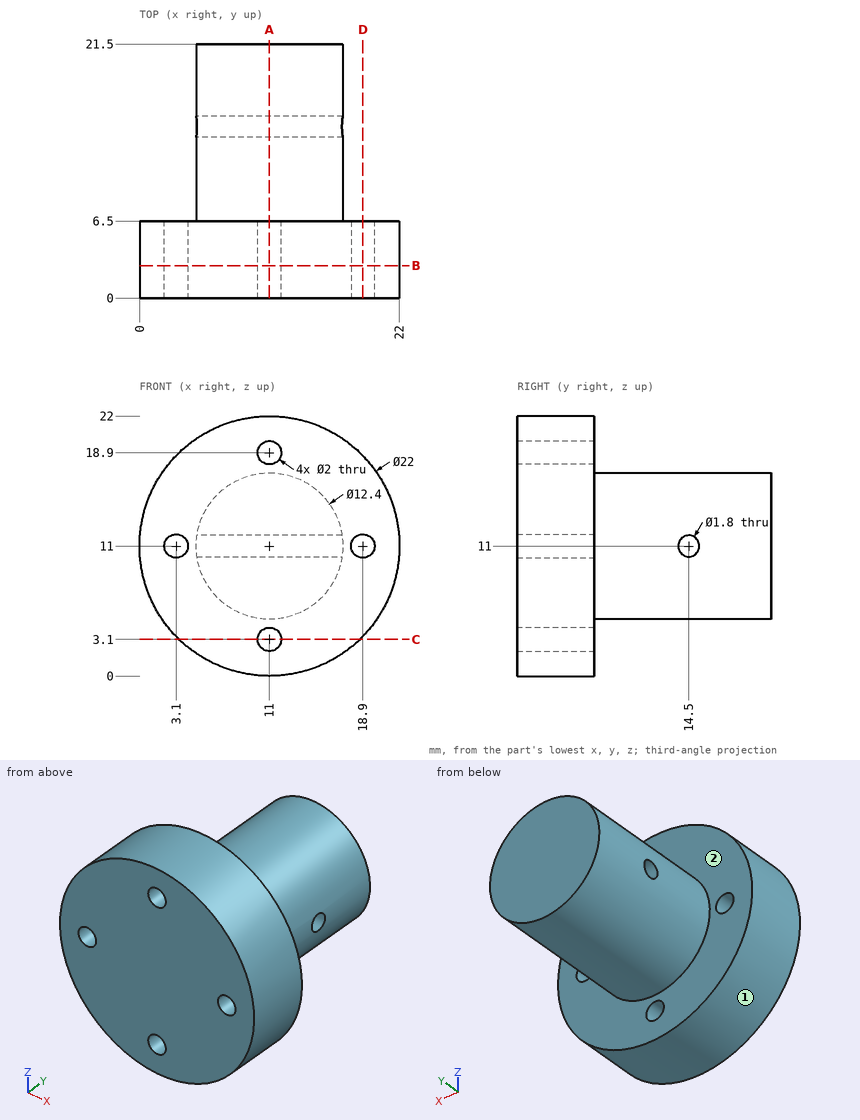
Design review of the part shown in the three views and the two pictorial views. Dimensions are in mm from the part's minimum x, y and z. A direction names the side the tool comes from. Round coordinates to 2 decimals unless told otherwise and drop trailing zeros. Order: outer loops, then holes, each group sorted by start corner. A loop starts at its lowest first (then second) coordinate and runs counter-clockwise, first axis right, second up.
Q1. We need section B-B, the plane y = 2.75. Give the boundary of the cut face in (x, z).
Findings below:
outline: circle Ø22 at (11, 11); hole circle Ø2 at (3.1, 11); hole circle Ø2 at (11, 3.1); hole circle Ø2 at (11, 18.9); hole circle Ø2 at (18.9, 11)
Q2. We need section A-A, the plane x = 11. Give the boundary of the cut face in (y, z), plus the area to 3 significant figures.
Findings below:
outline: (0, 0) - (6.5, 0) - (6.5, 2.1) - (0, 2.1) - close; (0, 4.1) - (6.5, 4.1) - (6.5, 4.8) - (21.5, 4.8) - (21.5, 17.2) - (6.5, 17.2) - (6.5, 17.9) - (0, 17.9) - close; (0, 19.9) - (6.5, 19.9) - (6.5, 22) - (0, 22) - close; hole circle Ø1.8 at (14.5, 11)
area: 300 mm2
Q3. Wall thickness on line 1 (Z direction, x = 10.75, y = 14.5); line 2 (Y direction, x = 6.25, z = 11); line 3 (Y direction, x = 13.75, z = 17.5): over which ranges is each line inside the solid? List them lowest first.
Findings below:
line 1: z = 4.81 to 10.1, 11.9 to 17.19
line 2: y = 0 to 13.6, 15.4 to 21.5
line 3: y = 0 to 6.5
Q4. Insertion check: P1, Ø10, axis at x = 5.5, y = 6, coming from the -Z side; P2, Ø1, axis at x = 10.5, y = 5, coming from the +Z side; P3, Ø4, axis at x = 17.5, y = 17, coming from the +Z side (3 decimals); P4, Ø1.6, axis at y = 14.5, z = 11, coming from the +X side. Each pin has a flat end and moves straight along its axis. Give the tip position at first contact, or say it passes through.
Findings below:
P1: stops at z = 0.01
P2: stops at z = 22
P3: stops at z = 15.265
P4: passes through
Q5. Machinability: for the marked faces 1 and 2, which of the approach directions +Z, -Z, +X, -X, +Y, -Y give a long, thin tool a straight path to every point of the face, cutting with its end or side? Answer none if there is none.
Findings below:
face 1: +Y, -Y
face 2: +Y
Q6. We need section C-C, the plane z = 3.1. Give the boundary of the cut face in (x, y), plus the area to 3 significant figures.
Findings below:
outline: (3.35, 0) - (10, 0) - (10, 6.5) - (3.35, 6.5) - close; (12, 0) - (18.65, 0) - (18.65, 6.5) - (12, 6.5) - close
area: 86.5 mm2
Q7. We need section D-D, the plane x = 18.9. Give the boundary of the cut face in (y, z), plus the area to 3 significant figures.
Findings below:
outline: (0, 3.35) - (6.5, 3.35) - (6.5, 10) - (0, 10) - close; (0, 12) - (6.5, 12) - (6.5, 18.65) - (0, 18.65) - close
area: 86.5 mm2
